```python
from build123d import *

# Parameters (mm, degrees)
F0_R     = 127
F1_DEPTH = 19.05
F2_R     = 3.81
F3_T     = -2.54


# Not quite as in the source:
# - a shell that OpenCascade refuses in one call is made with other operations: the cavity is built on its own and cut out


with BuildPart() as f1:
    # F0 (on Front) → F1 (new body)
    with BuildSketch(Plane.XZ):
        Circle(F0_R)
    extrude(amount=F1_DEPTH)

    # F2
    f2_edges = [f1.edges().sort_by_distance(p)[0] for p in [
        (-127, 0, 0),
        (-127, -19.05, 0),
    ]]
    fillet(f2_edges, radius=F2_R)

    # F3: a shell. OpenCascade refuses it in one call, so the cavity is built on its own and cut out:
    # the body offset inwards by the wall thickness, plus a prism from it out through each open face.
    f3_core = offset(f1.part, amount=F3_T, mode=Mode.PRIVATE)
    f3_exits = [f3_core.faces().sort_by_distance(p)[0] for p in [
        (0, -2.54, 0),
    ]]
    add(f3_core, mode=Mode.SUBTRACT)
    extrude(f3_exits, amount=-F3_T, mode=Mode.SUBTRACT)


solid = f1.part
```
Design review of the part built by this model. Coordinates are the model's own, in mm. A direction names the side the tool comes from. Round coordinates to 2 decimals unless told otherwise and drop trailing zeros. Write each loop counter-clockwise with the first axis right and the second up, starting at its lowest first coordinate (ties: lowest second). Pieces come first, ordered by that corner, then holes. Notation, with made-up numbers: (-31.5, 89.25) -> (17.5, 89.25) arc R23 cw to (17.5, 120.25) -> close; hole circle Ø7 at (78.25, -28). An arc over 180 degrees is marked (long way). Answer in a Markdown table with one row per item.
Q1. Draft analysis for pull direction Z (two halves, no side actions). For faces 1 (the face through (-27.53, -9.44, -123.98)), 2 (the face through (-2, -19.05, 2)), 3 (the face through (-2, -16.51, 2)), state which applies: +Z half, -Z half, draft (parallel to the pull), parting line (faces both ways), or undercut.
The answers:
| item | result |
|---|---|
| face 1 | parting line |
| face 2 | draft |
| face 3 | undercut |
Q2. Take a section at B-B, the plane z = 0. State the section outline as (x, y) points.
The answers:
| item | result |
|---|---|
| outline | (-127, -15.24) arc R3.81 ccw to (-123.19, -19.05) -> (123.19, -19.05) arc R3.81 ccw to (127, -15.24) -> (127, -3.81) arc R3.81 ccw to (123.19, 0) -> (123.19, -2.54) arc R1.27 cw to (124.46, -3.81) -> (124.46, -15.24) arc R1.27 cw to (123.19, -16.51) -> (-123.19, -16.51) arc R1.27 cw to (-124.46, -15.24) -> (-124.46, -3.81) arc R1.27 cw to (-123.19, -2.54) -> (-123.19, 0) arc R3.81 ccw to (-127, -3.81) -> close |
Q3. Take a section at C-C, the plane y = -9.5. State the section outline as (x, z) points, then the cut area to 3 significant figures.
The answers:
| item | result |
|---|---|
| outline | circle Ø254 at (0, 0); hole circle Ø248.92 at (0, 0) |
| area | 2,010 mm² |
Q4. Take a section at A-A, the plane x = 0. State the section outline as (y, z) points.
The answers:
| item | result |
|---|---|
| outline | (-19.05, -123.19) arc R3.81 ccw to (-15.24, -127) -> (-3.81, -127) arc R3.81 ccw to (0, -123.19) -> (-2.54, -123.19) arc R1.27 cw to (-3.81, -124.46) -> (-15.24, -124.46) arc R1.27 cw to (-16.51, -123.19) -> (-16.51, 123.19) arc R1.27 cw to (-15.24, 124.46) -> (-3.81, 124.46) arc R1.27 cw to (-2.54, 123.19) -> (0, 123.19) arc R3.81 ccw to (-3.81, 127) -> (-15.24, 127) arc R3.81 ccw to (-19.05, 123.19) -> close |
Q5. To check wall thickness, follow L1, parallel to Z at x = 0, y = -6.75; L2, parallel to Y at x = -64.5, z = -27. State the ranges of each line that lie inside material, in increasing order. Write a range as [from, to].
The answers:
| item | result |
|---|---|
| L1 | [-127, -124.46], [124.46, 127] |
| L2 | [-19.05, -16.51] |
Q6. For faces 4 (the face through (-26.71, -1.29, -120.26)), 5 (the face through (-26.98, -9.44, -121.5)), list the 3-axis set-ups (+Z, -Z, +X, -X, +Y, -Y) from which the entire face can be reached by the end or side of a thin tool; tool diameter is ignored.
The answers:
| item | result |
|---|---|
| face 4 | +Y |
| face 5 | none |
Q7. Clearance check with flat-ended pins moving along their axes: pin 1 Ø12 at (x, z) = (-71, -43) entering from +Y; pin 2 Ø5 at (y, z) = (-6, -61.5) entering from -X; pin 3 Ø5 at (y, z) = (-3.5, 73) entering from +X. State where each tip first meets the part, or that it passes through.
The answers:
| item | result |
|---|---|
| pin 1 | y = -16.51 |
| pin 2 | x = -112.46 |
| pin 3 | x = 105.63 |
